Here's the drawing with two shaded views (mm, measured from the low corner). I have some questions. A direction names the side the tool comes from. Round coordinates to 2 decimals unless told otherwise and drop trailing zeros. Write each loop counter-clockwise with the first axis right and the second up, starting at its lowest first coordinate (ties: lowest second). Pieces come first, ordered by that corner, then holes.
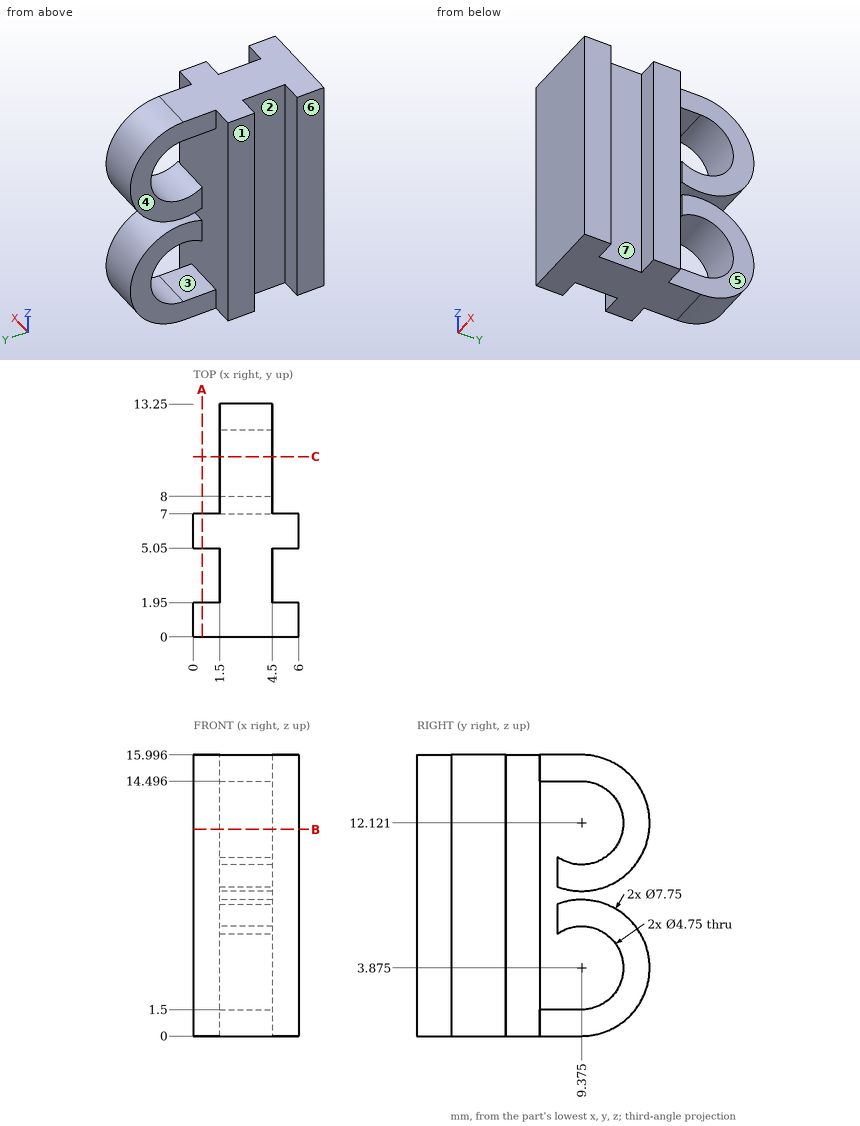
Q1. Imagine slicing it at A-A, the plane x = 0.5. Write out the boundary of the cut face in (y, z).
Q2. We'd pull the mould along Y, two halves only. Please class the marked faces 1, 2 and 3: pulls with the +Y half, pulls with the -Y half, needs draft (parallel to the pull), parting line crosses it, or undercut.
Q3. Imagine slicing it at C-C, the plane y = 10.25. Count the separate pieces of the cut face and the enclosed holes in it, then the cut area to 3 significant figures.
Q4. Imagine slicing it at B-B, the plane z = 11.75. Write out the boundary of the cut face in (x, y).
Q5. If I drill on L1, parallel to Y at x = 0.55, z = 5; L2, parallel to X at y = 12, z = 1.75; L3, parallel to Z at x = 3.35, y = 11.5 (1 decimal), over which ranges is the centre line in solid material (lowest first)?
Q6. On a 3-axis mill with a long thin cutter (end or side, diameter ignored), from which of +Z, -Z, +X, -X, +Y, -Y can I reach the whole of each face in a straight line? I mean the marked faces 4, 5, 6 and 7. Say none if no direction works.
Q7. I'm going to push flat-ended pins straight in: pin 1 Ø1 at (y, z) = (10, 8.5) entering from +X; pin 2 Ø2.5 at (y, z) = (3.5, 7) entering from -X; pin 3 Ø1.2 at (x, z) = (1, 10.5) entering from +Y. Where does each tip first touch, or does it pass through?
Results found:
1. outline: (0, 0) - (1.95, 0) - (1.95, 16) - (0, 16) - close; (5.05, 0) - (7, 0) - (7, 16) - (5.05, 16) - close
2. face 1: needs draft
2. face 2: undercut
2. face 3: undercut
3. separate pieces: 4
3. enclosed holes: 0
3. area: 18.8 mm2
4. outline: (0, 0) - (6, 0) - (6, 1.95) - (4.5, 1.95) - (4.5, 5.05) - (6, 5.05) - (6, 7) - (0, 7) - (0, 5.05) - (1.5, 5.05) - (1.5, 1.95) - (0, 1.95) - close; (1.5, 11.72) - (4.5, 11.72) - (4.5, 13.23) - (1.5, 13.23) - close
5. L1: y = 0 to 1.95, 5.05 to 7
5. L2: x = 1.5 to 4.5
5. L3: z = 0.6 to 2.8, 4.9 to 7.1, 8.9 to 11.1, 13.2 to 15.4
6. face 4: +Z, -Z, -X, +Y
6. face 5: +Z, -Z, +X, +Y
6. face 6: +Z, -Z, -X, +Y, -Y
6. face 7: +Z, -Z, +X
7. pin 1: stops at x = 4.5
7. pin 2: stops at x = 1.5
7. pin 3: stops at y = 13.03
